Can you work these out from the drawing? Everything is in mm from the part's minimum corner. A direction names the side the tool comes from. Round coordinates to 2 decimals unless told otherwise and drop trailing zeros. Order: outer loops, then holes, each group sorted by start corner. A loop starts at its lowest first (then second) coordinate and runs counter-clockwise, first axis right, second up. Notation, with made-up numbers: (23, 27.25) - (31, 27.25) arc R21 ccw to (31, 51.25) - close; hole circle Ø2 at (38.5, 49). An arc over 180 degrees is marked (long way). Write item = value, one per line.
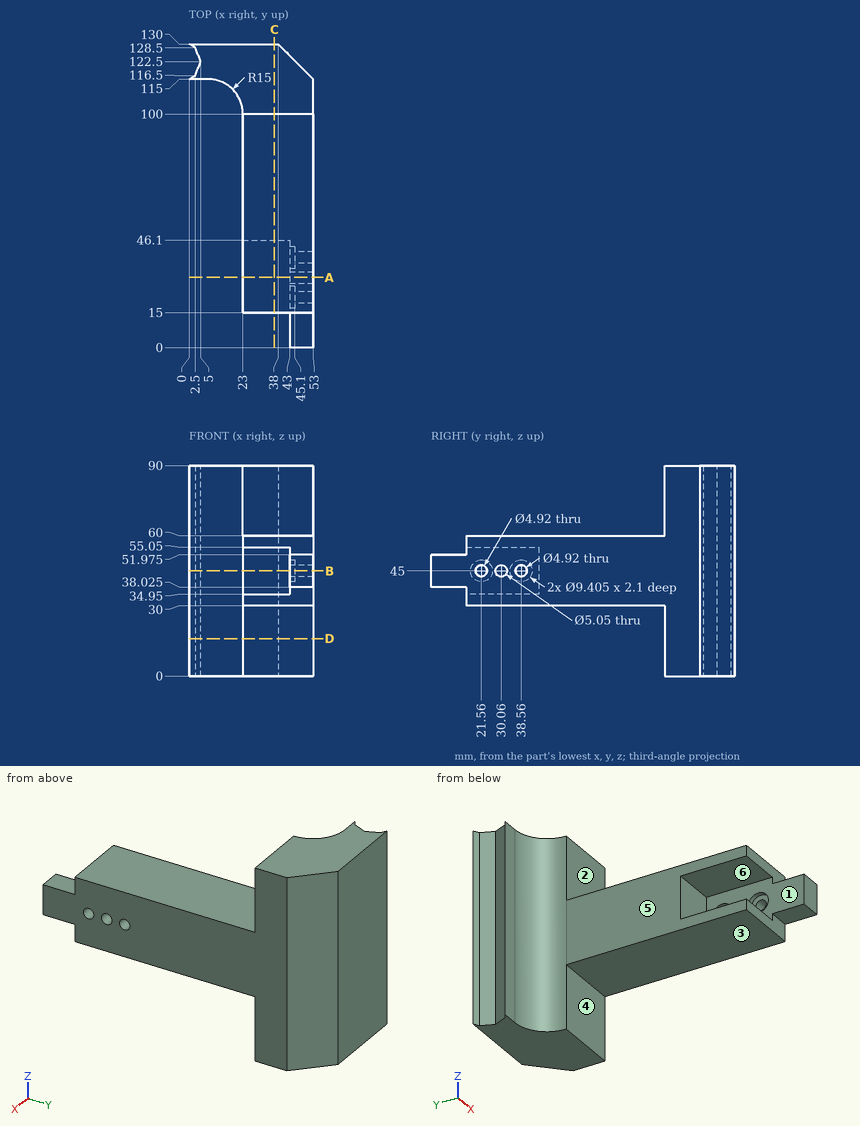
(1) If I drill on line 1 (Z direction, x = 44, y = 38); line 2 (Z direction, x = 35.5, y = 40.5); line 3 (X direction, y = 37.5, z = 52.5), over which ranges is the centre line in solid material (lowest first)? Write a range as from..to.
Computed:
line_1 = 30..40.33, 49.67..60
line_2 = 30..34.95, 55.05..60
line_3 = 43..53
(2) On a 3-axis mill with a long thin cutter (end or side, diameter ignored), from which of +Z, -Z, +X, -X, +Y, -Y can I reach the whole of each face in a straight line? I mean the marked faces 4, 5 and 6. Say none if no direction works.
Computed:
face_4 = -Z, +X, -X, -Y
face_5 = +Z, -Z, -X, -Y
face_6 = -X, -Y
(3) If we section it at A-A (y = 30.06): Write out the boundary of the cut face in (x, z) (3 decimals), plus the area to 4 significant figures.
Computed:
outline = (23, 30) - (53, 30) - (53, 42.475) - (43, 42.475) - (43, 34.95) - (23, 34.95) - close; (23, 55.05) - (43, 55.05) - (43, 47.525) - (53, 47.525) - (53, 60) - (23, 60) - close
area = 447.5 mm^2
(4) If we section it at D-D (z = 16): Write out the boundary of the cut face in (x, y).
Computed:
outline = (0, 115) - (8, 115) arc R15 cw to (23, 100) - (53, 100) - (53, 115) - (38, 130) - (0, 130) - (2.5, 128.5) - (5, 122.5) - (2.5, 116.5) - close
(5) If we section it at B-B (z = 45): State how many separate pieces and enclosed holes the cut face has, plus the area to 3 significant figures.
Computed:
separate_pieces = 4
enclosed_holes = 0
area = 3,040 mm^2
(6) Will these pins go through, and if not, where does the flat tip stop? P1, Ø24, axis at x = 44, y = 40.5, coming from the +Z side; P2, Ø6.5, axis at x = 42.5, z = 34.5, coming from the -Y side; P3, Ø8, axis at x = 44, y = 56, coming from the -Z side.
Computed:
P1 = 60
P2 = 15
P3 = 30
(7) If we section it at C-C (x = 36.5): Write out the boundary of the cut face in (y, z), plus the area to 3 significant figures.
Computed:
outline = (15, 30) - (100, 30) - (100, 0) - (130, 0) - (130, 90) - (100, 90) - (100, 60) - (15, 60) - (15, 55.05) - (46.1, 55.05) - (46.1, 34.95) - (15, 34.95) - close
area = 4,620 mm^2
(8) Thinking about a two-plate mould opening in Z: for the marked faces 1, 2 and 3, which applies, +Z half, -Z half, draft (parallel to the pull), parting line (faces both ways), or undercut?
Computed:
face_1 = undercut
face_2 = draft
face_3 = -Z half
